Here's how the part is built. I have some questions about the finished solid (model axes, mm). A direction names the side the tool comes from. Round coordinates to 2 decimals unless told otherwise and drop trailing zeros. Loops run counter-clockwise (first coordinate to the right, second up) from the corner with the lowest first, then second, coordinate; pieces in that order, holes last. Notation, with made-up numbers: (62, 68) - (100, 68) arc R7 cw to (100, 78) - close; hole circle Ø2 at (44, 16). An arc over 180 degrees is marked (long way). Answer as a JSON object with one key per item and string values. Group by question number.
1) If we mould it in two halves opening along X, with no side actions, what happens to faces 1 (the face through (-1, -17, 7.5)), 2 (the face through (-0.933, -0.982, 3.66)), 3 (the face through (17.359, 17.297, 1.014))? For each: pulls with the +X half, pulls with the -X half, needs draft (parallel to the pull), parting line crosses it, or undercut.
2) I want a section at D-D, the plane x = -7. Please give me the cut outline in (y, z), then the cut area to 3 significant figures.
3) I want a section at C-C, the plane z = 3. Please give me the cut outline in (x, y), then the cut area to 3 significant figures.
4) Will these pins go through, and if not, where does the flat tip stop? P1, Ø5.5, axis at y = -6.5, z = 10, coming from the +X side; P2, Ø1.5, axis at x = 9, y = 13.5, coming from the +Z side; P3, Ø10, axis at x = 0, z = 15.5, coming from the +Y side; P4, Ø1.5, axis at x = 6, z = 7.5, coming from the -Y side.
5) I want a section at B-B, the plane y = 15.25. Please give me the cut outline in (x, z) (3 decimals), then the cut area to 3 significant figures.
6) I want a section at A-A, the plane x = 16. Please give me the cut outline in (y, z).
7) Which directions (+Z, -Z, +X, -X, +Y, -Y) give clear straight access to the entire face, cutting with the end or side of a thin tool? Please do faces 4 (the face through (-6.736, 0.818, 9.364)), 5 (the face through (0, 18.5, 1)), 6 (the face through (6, -6.391, 1)).
8) If I drill on line 1 along X through (y, z) = (-11, 10.75); line 2 along Y through (x, z) = (15.25, 0.9) (3 decimals); line 3 along Z through (x, y) = (6, 15.5), over which ranges is the centre line in solid material (lowest first)? Write a range as [from, to].
from build123d import *

# Parameters (mm, degrees)
F0_W     = 37
F0_H     = 37
F0_R     = 1.575
F1_DEPTH = 2
F3_DEPTH = 26.25
F4_DEPTH = 24.25
F5_DEPTH = 14.75
F6_DEPTH = 12.75
F7_R     = 4
F8_W     = 1.5
F8_H     = 3
F9_DEPTH = 25


with BuildPart() as f1:
    # F0 (on Top) → F1 (new body)
    with BuildSketch(Plane.XY):
        Rectangle(F0_W, F0_H)
        with Locations((-15.25, -15.25)):
            Circle(F0_R, mode=Mode.SUBTRACT)
        with Locations((15.25, -15.25)):
            Circle(F0_R, mode=Mode.SUBTRACT)
        with Locations((-15.25, 15.25)):
            Circle(F0_R, mode=Mode.SUBTRACT)
        with Locations((15.25, 15.25)):
            Circle(F0_R, mode=Mode.SUBTRACT)
    extrude(amount=F1_DEPTH)

    # F2 (on face) → F3 (join)
    with BuildSketch(Plane.YZ.offset(18.5)):
        Polygon((-12.187941467, 17.9895313658), (-15.5, 7.5), (-1.5066505404, 2), (-0.4433530164, 5.3675409473), (2.1159649409, 13.4730879118), (-6.4663789039, 16.1829539842), (-6.6681133781, 15.5440461646), (-9.5288946597, 16.4473348554), (-9.3271601854, 17.086242675), align=None)
        Polygon((-18.5, 7.5), (-18.5, 2), (-1.5066505404, 2), (-15.5, 7.5), align=None)
        Polygon((-0.4433530164, 5.3675409473), (-1.5066505404, 2), (2.58314132, 2), (3.2756626496, 4.1932656492), align=None)
    extrude(amount=-F3_DEPTH)

    # F2 (on face) → F4 (cut)
    with BuildSketch(Plane.YZ.offset(18.5)):
        Polygon((-15.5, 7.5), (-1.5066505404, 2), (-0.4433530164, 5.3675409473), (2.1159649409, 13.4730879118), (-6.4663789039, 16.1829539842), (-6.6681133781, 15.5440461646), (-9.5288946597, 16.4473348554), (-9.3271601854, 17.086242675), (-12.187941467, 17.9895313658), align=None)
    extrude(amount=-F4_DEPTH, mode=Mode.SUBTRACT)

    # F2 (on face) → F5 (join)
    with BuildSketch(Plane.YZ.offset(18.5)):
        Polygon((-12.187941467, 17.9895313658), (-15.5, 7.5), (-1.5066505404, 2), (-0.4433530164, 5.3675409473), (2.1159649409, 13.4730879118), (-6.4663789039, 16.1829539842), (-6.6681133781, 15.5440461646), (-9.5288946597, 16.4473348554), (-9.3271601854, 17.086242675), align=None)
        Polygon((-18.5, 7.5), (-18.5, 2), (-1.5066505404, 2), (-15.5, 7.5), align=None)
        Polygon((-0.4433530164, 5.3675409473), (-1.5066505404, 2), (2.58314132, 2), (3.2756626496, 4.1932656492), align=None)
    extrude(amount=-F5_DEPTH)

    # F2 (on face) → F6 (cut)
    with BuildSketch(Plane.YZ.offset(18.5)):
        Polygon((-12.187941467, 17.9895313658), (-15.5, 7.5), (-1.5066505404, 2), (-0.4433530164, 5.3675409473), (2.1159649409, 13.4730879118), (-6.4663789039, 16.1829539842), (-6.6681133781, 15.5440461646), (-9.5288946597, 16.4473348554), (-9.3271601854, 17.086242675), align=None)
        Polygon((-18.5, 7.5), (-18.5, 2), (-1.5066505404, 2), (-15.5, 7.5), align=None)
        Polygon((-0.4433530164, 5.3675409473), (-1.5066505404, 2), (2.58314132, 2), (3.2756626496, 4.1932656492), align=None)
    extrude(amount=-F6_DEPTH, mode=Mode.SUBTRACT)

    # F7
    f7_edges = [f1.edges().sort_by_distance(p)[0] for p in [
        (18.5, -18.5, 1),
        (18.5, 18.5, 1),
        (-18.5, 18.5, 1),
        (-18.5, -18.5, 1),
    ]]
    fillet(f7_edges, radius=F7_R)

    # F8 (on face) → F9 (cut)
    with BuildSketch(Plane.XY.offset(2)):
        with Locations((-8.5, -7.8909632415)):
            Rectangle(F8_W, F8_H)
        with Locations((6.5, -7.8909632415)):
            Rectangle(F8_W, F8_H)
    extrude(amount=-F9_DEPTH, mode=Mode.SUBTRACT)


solid = f1.part
Outcome:
{
 "1": {"face 1": "needs draft", "face 2": "undercut", "face 3": "pulls with the +X half"},
 "2": {"outline": "(-18.5, 0) - (18.5, 0) - (18.5, 2) - (2.58, 2) - (3.28, 4.19) - (-0.44, 5.37) - (2.12, 13.47) - (-6.47, 16.18) - (-6.67, 15.54) - (-9.53, 16.45) - (-9.33, 17.09) - (-12.19, 17.99) - (-15.5, 7.5) - (-18.5, 7.5) - close", "area": "311 mm^2"},
 "3": {"outline": "(-7.75, -18.5) - (5.75, -18.5) - (5.75, 2.9) - (-7.75, 2.9) - close; hole (-5.75, -4.05) - (3.75, -4.05) - (3.75, -1.19) - (-5.75, -1.19) - close", "area": "262 mm^2"},
 "4": {"P1": "x = 5.75", "P2": "z = 2", "P3": "y = 2.12", "P4": "y = -18.5"},
 "5": {"outline": "(-18.429, 0) - (-16.825, 0) - (-16.825, 2) - (-18.429, 2) - close; (-13.675, 0) - (13.675, 0) - (13.675, 2) - (-13.675, 2) - close; (16.825, 0) - (18.429, 0) - (18.429, 2) - (16.825, 2) - close", "area": "61.1 mm^2"},
 "6": {"outline": "(-18.21, 0) - (-16.63, 0) - (-16.63, 2) - (-18.21, 2) - close; (-13.87, 0) - (13.87, 0) - (13.87, 2) - (-13.87, 2) - close; (16.63, 0) - (18.21, 0) - (18.21, 2) - (16.63, 2) - close"},
 "7": {"face 4": "+X, -X, +Y", "face 5": "+Z, -Z, +X, -X, +Y", "face 6": "+Z, -Z"},
 "8": {"line 1": "[-7.75, -5.75], [3.75, 5.75]", "line 2": "[-18.429, -16.825], [-13.675, 13.675], [16.825, 18.429]", "line 3": "[0, 2]"}
}
